```python
from build123d import *

# Parameters (mm, degrees)
EXTRUDE_THIN1_DEPTH     = 3
BOSS_EXTRUDE1_DEPTH     = 1
EXTRUDE_THIN2_OUTLINE_W = 18.914434681
EXTRUDE_THIN2_OUTLINE_H = 1
EXTRUDE_THIN2_DEPTH     = 10
SKETCH4_4_W             = 1
SKETCH4_4_H             = 22.9
EXTRUDE_THIN3_DEPTH     = 10
SKETCH5_R               = 5.249261594
SKETCH5_R_2             = 4.249261594
EXTRUDE_THIN4_DEPTH     = 10
SKETCH5_4_R             = 1.494593426
SKETCH5_4_R_2           = 1.433178879
CUT_EXTRUDE1_DEPTH      = 10
EXTRUDE_THIN5_START     = 12
EXTRUDE_THIN5_DEPTH     = 4


# Read off the part's stored shape, not the designer's step: Extrude-Thin1, Extrude-Thin2
with BuildPart() as part:
    # Extrude-Thin1 outline → Extrude-Thin1 (new body)
    with BuildSketch(Plane.XY):
        with BuildLine():
            Line((-2.95492513, -17.245283727), (-13.072339205, -17.798123277))
            ThreePointArc((-13.072339205, -17.798123277), (-22.52672937, -27.783227678), (-13.072339205, -37.76833208))
            Line((-13.072339205, -37.76833208), (-2.95492513, -38.32117163))
            ThreePointArc((-2.95492513, -38.32117163), (12.97327063, -27.783227679), (-2.95492513, -17.245283727))
        make_face()
        with BuildLine():
            ThreePointArc((-12.635851337, -29.780248558), (-14.52672937, -27.783227678), (-12.635851337, -25.786206798))
            Line((-12.635851337, -25.786206798), (-0.685801573, -25.133227678))
            ThreePointArc((-0.685801573, -25.133227678), (4.97327063, -27.783227678), (-0.685801573, -30.433227678))
            Line((-0.685801573, -30.433227678), (-12.635851337, -29.780248558))
        make_face(mode=Mode.SUBTRACT)
    extrude(amount=EXTRUDE_THIN1_DEPTH)

    # Sketch3 → Boss-Extrude1 (add)
    with BuildSketch(Plane.XY.offset(3)):
        with BuildLine():
            Line((-2.95492513, -17.245283727), (-13.072339205, -17.798123277))
            ThreePointArc((-13.072339205, -17.798123277), (-22.52672937, -27.783227678), (-13.072339205, -37.76833208))
            Line((-13.072339205, -37.76833208), (-2.95492513, -38.32117163))
            ThreePointArc((-2.95492513, -38.32117163), (12.97327063, -27.783227678), (-2.95492513, -17.245283727))
        make_face()
    extrude(amount=BOSS_EXTRUDE1_DEPTH)

    # Extrude-Thin2 outline → Extrude-Thin2 (add)
    with BuildSketch(Plane.XY.offset(4)):
        with Locations((3.516053289, -27.783227678)):
            Rectangle(EXTRUDE_THIN2_OUTLINE_W, EXTRUDE_THIN2_OUTLINE_H)
    extrude(amount=EXTRUDE_THIN2_DEPTH)

    # Sketch4<4> → Extrude-Thin3 (add)
    with BuildSketch(Plane.XY.offset(4)):
        with Locations((1.52327063, -27.783227678)):
            Rectangle(SKETCH4_4_W, SKETCH4_4_H)
        Polygon((12.97327063, -27.283227678), (-2.95492513, -27.283227678), (-5.941164051, -27.283227678), (-5.941164051, -28.283227678), (-2.95492513, -28.283227678), (12.97327063, -28.283227678), align=None)
    extrude(amount=EXTRUDE_THIN3_DEPTH)

    # Sketch5 → Extrude-Thin4 (add)
    # profile 1 of 2: a face of its own
    with BuildSketch(Plane(origin=(2.02327063, 0, 0), x_dir=(0, 0, -1), z_dir=(1, 0, 0))):
        with Locations((-8.640362386, -33.615627273)):
            Circle(SKETCH5_R)
        with Locations((-8.640362386, -33.615627273)):
            Circle(SKETCH5_R_2, mode=Mode.SUBTRACT)
    # profile 2 of 2: a face of its own
    with BuildSketch(Plane(origin=(2.02327063, 0, 0), x_dir=(0, 0, -1), z_dir=(1, 0, 0))):
        with Locations((-8.640362386, -21.950828084)):
            Circle(SKETCH5_R)
        with Locations((-8.640362386, -21.950828084)):
            Circle(SKETCH5_R_2, mode=Mode.SUBTRACT)
    extrude(amount=EXTRUDE_THIN4_DEPTH)

    # Sketch5<4> → Cut-Extrude1 (cut)
    with BuildSketch(Plane(origin=(2.02327063, 0, 0), x_dir=(0, 0, -1), z_dir=(1, 0, 0))):
        with Locations(Location((-8.640362386, -36.205301228, 0), (0, 0, 90))):
            Circle(SKETCH5_4_R)
        with Locations(Location((-8.640362386, -30.946846255, 0), (0, 0, 90))):
            Circle(SKETCH5_4_R_2)
        with Locations(Location((-8.640362386, -24.619609101, 0), (0, 0, 90))):
            Circle(SKETCH5_4_R_2)
        with Locations(Location((-8.640362386, -19.361154128, 0), (0, 0, 90))):
            Circle(SKETCH5_4_R)
    extrude(amount=-CUT_EXTRUDE1_DEPTH, mode=Mode.SUBTRACT)

    # Sketch6 → Extrude-Thin5 (add)
    with BuildSketch(Plane.ZY.offset(5.941164051).offset(EXTRUDE_THIN5_START)):
        with BuildLine():
            Line((4, -25.018913287), (8.306214493, -25.018913287))
            ThreePointArc((8.306214493, -25.018913287), (11.024963262, -27.737662056), (8.306214493, -30.456410826))
            Line((8.306214493, -30.456410826), (4, -30.456410826))
            Line((4, -30.456410826), (4, -29.456410826))
            Line((4, -29.456410826), (8.306214493, -29.456410826))
            ThreePointArc((8.306214493, -29.456410826), (10.024963262, -27.737662056), (8.306214493, -26.018913287))
            Line((8.306214493, -26.018913287), (4, -26.018913287))
            Line((4, -26.018913287), (4, -25.018913287))
        make_face()
    extrude(amount=EXTRUDE_THIN5_DEPTH)


solid = part.part
```
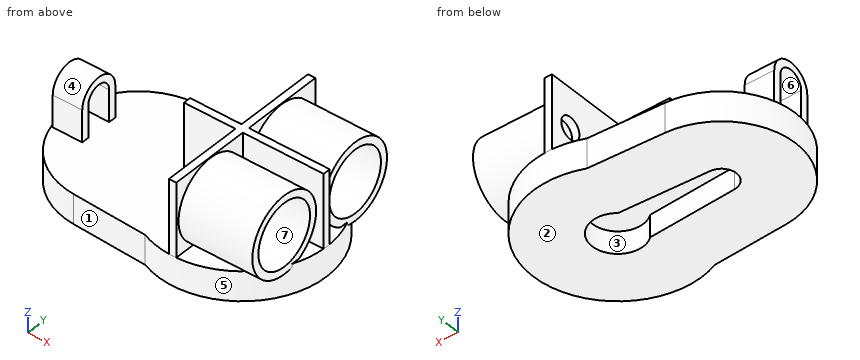
Source: CAD feature listing. Evaluate the final solid. Frame: model axes, mm. Face numbers are marked on the shaded views. A direction names the side the tool comes from. Round coordinates to 2 decimals unless told otherwise and drop trailing zeros. Order: outer loops, then holes, each group sorted by start corner. A loop starts at its lowest first (then second) coordinate and runs counter-clockwise, first axis right, second up. Notation, with made-up numbers: (-31, -19.75) -> (24, -19.75) arc R31 cw to (24, 14.25) -> close; hole circle Ø4 at (2, 2). An arc over 180 degrees is marked (long way). One line per item, written item: value. Start each with the question number.
Q1. Draft query along X for the marked faces 1, 2 and 3. Return one class per face: pulls with the +X half, pulls with the -X half, needs draft (parallel to the pull), parting line crosses it, or undercut.
Q2. Section query B-B (y = -37.25). Return the cut outline in (x, z), plus the area to 3 significant figures.
Q3. Section query A-A (z = 2.5). Return the cut outline in (x, y).
Q4. Section query C-C (x = 10.5). Return the cut outline in (y, z), plus the area to 3 significant figures.
Q5. Pin query (flat end, axial travel): pin 1 (2 mm diameter, centred on x = -2.5, y = -28, fed in from -Z); pin 2 (2 mm diameter, centred on x = -3.5, z = 10.5, fed in from +Y); pin 3 (6 mm diameter, centred on y = -34.5, z = 11, fed in from +X). Return the tip coordinate at first contact, or that it passes through.
Q6. Access query for the marked faces 4, 5, 6 and 7. Directions: +Z, -Z, +X, -X, +Y, -Y. A direction counts if a zero-diameter tool reaches every point of the face in a straight line with its end or side. Return the directions, or none.
Q7. Section query D-D (y = -32.75). Return the cut outline in (x, z), plus the area to 3 significant figures.
Q8. Material intervals for probe 1 along Y at (x, z) = (3, 11); probe 2 along Y at (x, z) = (9, 12.5); probe 3 along Z at (x, y) = (-20, -27.75), sorted ascending.
Findings below:
1. face 1: pulls with the -X half
1. face 2: needs draft
1. face 3: undercut
2. outline: (-15.75, 0) -> (7.96, 0) -> (7.96, 4) -> (2.02, 4) -> (2.02, 4.85) -> (12.02, 4.85) -> (12.02, 6.44) -> (2.02, 6.44) -> (2.02, 7.57) -> (1.02, 7.57) -> (1.02, 4) -> (-15.75, 4) -> close; (1.02, 9.71) -> (2.02, 9.71) -> (2.02, 10.84) -> (12.02, 10.84) -> (12.02, 12.43) -> (2.02, 12.43) -> (2.02, 14) -> (1.02, 14) -> close
2. area: 134 mm²
3. outline: (-13.07, -37.77) -> (-2.95, -38.32) arc R11.45 ccw (long way) to (-2.95, -17.25) -> (-13.07, -17.8) arc R10 ccw to start; hole (-12.64, -29.78) -> (-0.69, -30.43) arc R3.45 ccw (long way) to (-0.69, -25.13) -> (-12.64, -25.79) arc R2 ccw to start
4. outline: (-34.89, 0) -> (-20.68, 0) -> (-20.68, 3.55) arc R5.25 ccw (long way) to (-24.4, 4) -> (-27.28, 4) -> (-27.28, 14) -> (-28.28, 14) -> (-28.28, 4) -> (-31.16, 4) arc R5.25 ccw (long way) to (-34.89, 3.55) -> close; hole circle Ø8.5 at (-33.62, 8.64); hole circle Ø8.5 at (-21.95, 8.64)
4. area: 123 mm²
5. pin 1: z = 3
5. pin 2: y = -27.28
5. pin 3: x = 12.02
6. face 4: +Z, -X
6. face 5: -Z
6. face 6: -X
6. face 7: +X
7. outline: (-21.21, 0) -> (11.84, 0) -> (11.84, 3.46) -> (12.02, 3.46) -> (12.02, 4.48) -> (2.02, 4.48) -> (2.02, 12.8) -> (12.02, 12.8) -> (12.02, 13.82) -> (2.02, 13.82) -> (2.02, 14) -> (1.02, 14) -> (1.02, 4) -> (-21.21, 4) -> close
7. area: 157 mm²
8. probe 1: -38.3 to -37.15, -30.08 to -28.93, -28.28 to -27.28, -26.64 to -25.48, -18.42 to -17.26
8. probe 2: -37.17 to -35.39, -31.84 to -30.06, -28.28 to -27.28, -25.51 to -23.73, -20.17 to -18.39
8. probe 3: 0 to 4, 10.02 to 11.02
